```python
from build123d import *

# Parameters (mm, degrees)
EXTRUDE_1_DEPTH     = 20
SKETCH_3_R          = 1.5
CUT_EXTRUDE_1_DEPTH = 20
SKETCH_4_R          = 5
CUT_EXTRUDE_2_DEPTH = 20


with BuildPart() as part:
    # 草图1 → 凸台-拉伸1 (new body)
    with BuildSketch(Plane.XY):
        Polygon((0, 0), (25, 0), (25, 2), (2, 2), (2, 38), (0, 38), align=None)
    extrude(amount=EXTRUDE_1_DEPTH)

    # 草图3 → 切除-拉伸1 (cut)
    with BuildSketch(Plane(origin=(0, 2, 0), x_dir=(1, 0, 0), z_dir=(0, 1, 0))):
        with Locations(Location((17, -5, 0), (0, 0, 180))):
            Circle(SKETCH_3_R)
        with Locations(Location((17, -15, 0), (0, 0, 180))):
            Circle(SKETCH_3_R)
        with Locations(Location((7, -5, 0), (0, 0, 180))):
            Circle(SKETCH_3_R)
        with Locations(Location((7, -15, 0), (0, 0, 180))):
            Circle(SKETCH_3_R)
    extrude(amount=-CUT_EXTRUDE_1_DEPTH, mode=Mode.SUBTRACT)

    # 草图4 → 切除-拉伸2 (cut)
    with BuildSketch(Plane(origin=(2, 0, 0), x_dir=(0, 0, -1), z_dir=(1, 0, 0))):
        with Locations(Location((-10, 20, 0), (0, 0, 90))):
            Circle(SKETCH_4_R)
    extrude(amount=-CUT_EXTRUDE_2_DEPTH, mode=Mode.SUBTRACT)


solid = part.part
```
Read the model definition and answer for the solid it produces. Units are mm, in the model's axes. A direction names the side the tool comes from. Coordinates: 2 decimals unless noted, no trailing zeros. Loops run counter-clockwise (first coordinate to the right, second up) from the corner with the lowest first, then second, coordinate; pieces in that order, holes last.
(1) The part is cut by section A-A (x = 7). Determine the outline of the cut face in (y, z).
Solution:
outline: (0, 0) - (2, 0) - (2, 3.5) - (0, 3.5) - close; (0, 6.5) - (2, 6.5) - (2, 13.5) - (0, 13.5) - close; (0, 16.5) - (2, 16.5) - (2, 20) - (0, 20) - close
(2) A tool of negligible diameter and unlimited length cuts with its end or side. For faces 4 (the face through (14, 2, 10)), 5 (the face through (1, 38, 10)), from which of +Z, -Z, +X, -X, +Y, -Y can it reach the whole face along a straight path? Write none if from no direction.
Solution:
face 4: +Z, -Z, +X, +Y
face 5: +Z, -Z, +X, -X, +Y
(3) The mould has two halves that part along Z. Classify faces 1 (the face through (8.5, 1.01, 5.07)), 2 (the face through (1, 13, 20)), 3 (the face through (25, 1, 10)): released by +Z, released by -Z, zero draft, split by the parting line, or undercut.
Solution:
face 1: undercut
face 2: released by +Z
face 3: zero draft
(4) The part is cut by section C-C (y = 20). Determine the outline of the cut face in (x, z).
Solution:
outline: (0, 0) - (2, 0) - (2, 5) - (0, 5) - close; (0, 15) - (2, 15) - (2, 20) - (0, 20) - close
(5) The part is cut by section B-B (z = 10). Determine the outline of the cut face in (x, y).
Solution:
outline: (0, 0) - (25, 0) - (25, 2) - (2, 2) - (2, 15) - (0, 15) - close; (0, 25) - (2, 25) - (2, 38) - (0, 38) - close
(6) The part is cut by section D-D (z = 7.5). Determine the outline of the cut face in (x, y).
Solution:
outline: (0, 0) - (25, 0) - (25, 2) - (2, 2) - (2, 15.67) - (0, 15.67) - close; (0, 24.33) - (2, 24.33) - (2, 38) - (0, 38) - close
(7) Flat-ended cylindrical pins translate along their axes: pin 1 Ø1 at (y, z) = (26.5, 4.5) entering from +X; pin 2 Ø6 at (x, z) = (21.5, 12.5) entering from +Y. Find the tip coordinate at first contact, or state that the pin passes through.
Solution:
pin 1: stops at x = 2
pin 2: stops at y = 2
(8) Consider line 1 along Z through (x, y) = (7, 0.7); line 2 along Z through (x, y) = (0.4, 20); line 3 along X through (y, z) = (7.5, 9.75). Determine where each line is inside the solid, lowest interval first.
Solution:
line 1: z = 0 to 3.5, 6.5 to 13.5, 16.5 to 20
line 2: z = 0 to 5, 15 to 20
line 3: x = 0 to 2
